Verification items for the finished model (mm, model axes). Round coordinates to 2 decimals unless told otherwise and drop trailing zeros. Write each loop counter-clockwise with the first axis right and the second up, starting at its lowest first coordinate (ties: lowest second). Pieces come first, ordered by that corner, then holes. Notation, with made-up numbers: (67.5, 10.5) -> (92.5, 10.5) arc R17 cw to (92.5, 25.5) -> close; hole circle Ø3 at (76.5, 60.25). An arc over 180 degrees is marked (long way). Answer as a JSON object with one key per item and string values. Group by question number.
(1) Sectioned sample at B-B on x = -38. Record the cut outline in (y, z).
(2) Draft check along Y on faces 1 (the face through (-38.202, 63.537, 0.493)), 2 (the face through (-0.15, -64.737, 0.493)), 3 (the face through (-1, 1, 0)), 4 (the face through (-24.202, 63.537, 0.493)). Enter one of: released by +Y, released by -Y, zero draft, split by the parting line, or undercut.
(3) Sectioned sample at A-A on y = 62. Record the cut outline in (x, z).
(4) Sectioned sample at C-C on x = -0.5. Record the cut outline in (y, z).
(5) Gauge pin test, flat end, axial feed: pin 1 Ø3 at (x, y) = (-38, 62) entering from +Z. Record the tip position at first contact, or that the pin passes through.
(6) Scan lines: L1, parallel to Y at x = 24.5, z = 0.85; L2, parallel to Y at x = 25, z = 0.1. Record each from-to range of solid material in increasing order. Write a range as from..to.
```python
from build123d import *

# Parameters (mm, degrees)
SKETCH_1_R      = 1.55
EXTRUDE_1_DEPTH = 1


with BuildPart() as part:
    # 草图1 → 凸台-拉伸1 (new body)
    with BuildSketch(Plane.XY):
        with BuildLine():
            Line((8.920204993, -71.5), (52.5, -71.5))
            Line((52.5, -71.5), (52.5, 71.5))
            Line((52.5, 71.5), (-52.5, 71.5))
            Line((-52.5, 71.5), (-52.5, -71.5))
            Line((-52.5, -71.5), (-8.920204993, -71.5))
            ThreePointArc((-8.920204993, -71.5), (-8.315996588, -71.296826332), (-7.957306659, -70.769864407))
            ThreePointArc((-7.957306659, -70.769864407), (0, -64.736088455), (7.957306659, -70.769864407))
            ThreePointArc((7.957306659, -70.769864407), (8.315996588, -71.296826332), (8.920204993, -71.5))
        make_face()
        with Locations((-38, 62)):
            Circle(SKETCH_1_R, mode=Mode.SUBTRACT)
        with Locations((-24, 62)):
            Circle(SKETCH_1_R, mode=Mode.SUBTRACT)
        with Locations((24, 62)):
            Circle(SKETCH_1_R, mode=Mode.SUBTRACT)
        with Locations((38, 62)):
            Circle(SKETCH_1_R, mode=Mode.SUBTRACT)
    extrude(amount=EXTRUDE_1_DEPTH)


solid = part.part
```
Computed values:
{
 "1": {"outline": "(-71.5, 0) -> (60.45, 0) -> (60.45, 1) -> (-71.5, 1) -> close; (63.55, 0) -> (71.5, 0) -> (71.5, 1) -> (63.55, 1) -> close"},
 "2": {"face 1": "undercut", "face 2": "released by -Y", "face 3": "zero draft", "face 4": "undercut"},
 "3": {"outline": "(-52.5, 0) -> (-39.55, 0) -> (-39.55, 1) -> (-52.5, 1) -> close; (-36.45, 0) -> (-25.55, 0) -> (-25.55, 1) -> (-36.45, 1) -> close; (-22.45, 0) -> (22.45, 0) -> (22.45, 1) -> (-22.45, 1) -> close; (25.55, 0) -> (36.45, 0) -> (36.45, 1) -> (25.55, 1) -> close; (39.55, 0) -> (52.5, 0) -> (52.5, 1) -> (39.55, 1) -> close"},
 "4": {"outline": "(-64.75, 0) -> (71.5, 0) -> (71.5, 1) -> (-64.75, 1) -> close"},
 "5": {"pin 1": "through"},
 "6": {"L1": "-71.5..60.53, 63.47..71.5", "L2": "-71.5..60.82, 63.18..71.5"}
}
